```python
from build123d import *

# Parameters (mm, degrees)
SKETCH_1_W          = 45
SKETCH_1_H          = 9
EXTRUDE_1_DEPTH     = 6
HOLE_WIZARD_M3_1_D  = 2.5
CUT_EXTRUDE_1_DEPTH = 47.281745862


with BuildPart() as part:
    # 草图1 → 凸台-拉伸1 (new body)
    with BuildSketch(Plane(origin=(0, 0, 0), x_dir=(1, 0, 0), z_dir=(0, 1, 0))):
        with Locations((22.5, 4.5)):
            Rectangle(SKETCH_1_W, SKETCH_1_H)
    extrude(amount=EXTRUDE_1_DEPTH)

    # M3 螺纹孔1 (through all)
    with Locations(Plane(origin=(0, 6, 0), x_dir=(1, 0, 0), z_dir=(0, 1, 0))):
        with Locations((2.5, 4.5), (8.5, 4.5), (36.5, 4.5), (42.5, 4.5)):
            Hole(HOLE_WIZARD_M3_1_D / 2)

    # 草图4 → 切除-拉伸1 (cut, through all)
    with BuildSketch(Plane.XY):
        with BuildLine():
            ThreePointArc((21.321428571, 2.072115639), (22.5, 1.5), (23.678571429, 2.072115639))
            ThreePointArc((23.678571429, 2.072115639), (28.5, 3), (23.678571429, 3.927884361))
            ThreePointArc((23.678571429, 3.927884361), (22.5, 4.5), (21.321428571, 3.927884361))
            ThreePointArc((21.321428571, 3.927884361), (16.5, 3), (21.321428571, 2.072115639))
        make_face()
    extrude(amount=-CUT_EXTRUDE_1_DEPTH, mode=Mode.SUBTRACT)


solid = part.part
```
Source: CAD feature listing. Evaluate the final solid. Frame: model axes, mm. A direction names the side the tool comes from. Give positions to 0.01 mm unless a question says otherwise; leave off trailing zeros. Order: outer loops, then holes, each group sorted by start corner. A loop starts at its lowest first (then second) coordinate and runs counter-clockwise, first axis right, second up.
(1) Pull-direction query (X, two-part tool) for faces 3 (the face through (37.49, 2.96, -3.74)), 4 (the face through (22, 1, -9)), 5 (the face through (45, 3, -4)); classes: +X half, -X half, draft (parallel to the pull), parting line (faces both ways), or undercut.
(2) Access query for faces 1 (the face through (22, 0, -5)), 2 (the face through (22.5, 4.5, -4.4)). Directions: +Z, -Z, +X, -X, +Y, -Y. A direction counts if a zero-diameter tool reaches every point of the face in a straight line with its end or side. Return the directions, or none.
(3) Section query C-C (z = -5). Return the cut outline in (x, y).
(4) Section query B-B (x = 26). Return the cut outline in (y, z).
(5) Material intervals for line 1 along Y through (x, z) = (21, -2); line 2 along Z through (x, y) = (36.5, 4.5); line 3 along X through (y, z) = (4.35, -1), sorted ascending.
(6) Section query A-A (y = 3). Return the cut outline in (x, z).
(7) Section query D-D (y = 1.1). Return the cut outline in (x, z), plus the area to 3 significant figures.
Outcome:
1. face 3: undercut
1. face 4: draft
1. face 5: +X half
2. face 1: +Z, -Z, +X, -X, -Y
2. face 2: +Z, -Z
3. outline: (0, 0) - (1.35, 0) - (1.35, 6) - (0, 6) - close; (3.65, 0) - (7.35, 0) - (7.35, 6) - (3.65, 6) - close; (9.65, 0) - (35.35, 0) - (35.35, 6) - (9.65, 6) - close; (37.65, 0) - (41.35, 0) - (41.35, 6) - (37.65, 6) - close; (43.65, 0) - (45, 0) - (45, 6) - (43.65, 6) - close; hole (21.32, 2.07) arc R1.5 ccw to (23.68, 2.07) arc R2.5 ccw (long way) to (23.68, 3.93) arc R1.5 ccw to (21.32, 3.93) arc R2.5 ccw (long way) to start
4. outline: (0, -9) - (0.5, -9) - (0.5, 0) - (0, 0) - close; (5.5, -9) - (6, -9) - (6, 0) - (5.5, 0) - close
5. line 1: y = 0 to 1.5, 4.5 to 6
5. line 2: z = -9 to -5.75, -3.25 to 0
5. line 3: x = 0 to 16.9, 21.1 to 21.85, 23.15 to 23.9, 28.1 to 45
6. outline: (0, -9) - (16.5, -9) - (16.5, 0) - (0, 0) - close; (28.5, -9) - (45, -9) - (45, 0) - (28.5, 0) - close; hole circle Ø2.5 at (2.5, -4.5); hole circle Ø2.5 at (8.5, -4.5); hole circle Ø2.5 at (36.5, -4.5); hole circle Ø2.5 at (42.5, -4.5)
7. outline: (0, -9) - (17.38, -9) - (17.38, 0) - (0, 0) - close; (20.62, -9) - (24.38, -9) - (24.38, 0) - (20.62, 0) - close; (27.62, -9) - (45, -9) - (45, 0) - (27.62, 0) - close; hole circle Ø2.5 at (2.5, -4.5); hole circle Ø2.5 at (8.5, -4.5); hole circle Ø2.5 at (36.5, -4.5); hole circle Ø2.5 at (42.5, -4.5)
7. area: 327 mm2
